```python
from build123d import *
from build123d.topology import SkipClean

# Parameters (mm, degrees)
SKETCH1_R           = 100
SKETCH1_R_2         = 50
BOSS_EXTRUDE3_DEPTH = 30
BOSS_EXTRUDE4_DEPTH = 10


with BuildPart() as part:
    # Sketch1 → Boss-Extrude3 (new body)
    # profile 1 of 16: a face of its own
    with SkipClean():  # the faces are left unmerged after this step: merging them gives an invalid solid
        with BuildSketch(Plane(origin=(0, 0, 0), x_dir=(1, 0, 0), z_dir=(0, 1, 0))):
            Circle(SKETCH1_R)
            with Locations(Location((0, 0, 0), (0, 0, 270))):
                Circle(SKETCH1_R_2, mode=Mode.SUBTRACT)
        # profile 2 of 16: a face of its own
        with BuildSketch(Plane(origin=(0, 0, 0), x_dir=(1, 0, 0), z_dir=(0, 1, 0))):
            with BuildLine():
                ThreePointArc((-15, 52.915026221), (0, 55), (15, 52.915026221))
                Line((15, 52.915026221), (15, 98.868599666))
                ThreePointArc((15, 98.868599666), (0, 100), (-15, 98.868599666))
                Line((-15, 98.868599666), (-15, 52.915026221))
            make_face()
        # profile 3 of 16: a face of its own
        with BuildSketch(Plane(origin=(0, 0, 0), x_dir=(1, 0, 0), z_dir=(0, 1, 0))):
            with BuildLine():
                ThreePointArc((-15, 47.696960071), (-7.587884964, 49.420886291), (0, 50))
                ThreePointArc((0, 50), (7.587884964, 49.420886291), (15, 47.696960071))
                Line((15, 47.696960071), (15, 52.915026221))
                ThreePointArc((15, 52.915026221), (0, 55), (-15, 52.915026221))
                Line((-15, 52.915026221), (-15, 47.696960071))
            make_face()
        # profile 4 of 16: a face of its own
        with BuildSketch(Plane(origin=(0, 0, 0), x_dir=(1, 0, 0), z_dir=(0, 1, 0))):
            with BuildLine():
                ThreePointArc((-15, 98.868599666), (0, 100), (15, 98.868599666))
                Line((15, 98.868599666), (15, 115))
                ThreePointArc((15, 115), (13.535533906, 118.535533906), (10, 120))
                Line((10, 120), (-10, 120))
                ThreePointArc((-10, 120), (-13.535533906, 118.535533906), (-15, 115))
                Line((-15, 115), (-15, 98.868599666))
            make_face()
        # profile 5 of 16: a face of its own
        with BuildSketch(Plane(origin=(0, 0, 0), x_dir=(1, 0, 0), z_dir=(0, 1, 0))):
            with BuildLine():
                ThreePointArc((-98.868599666, -15), (-100, 0), (-98.868599666, 15))
                Line((-98.868599666, 15), (-115, 15))
                ThreePointArc((-115, 15), (-118.535533906, 13.535533906), (-120, 10))
                Line((-120, 10), (-120, -10))
                ThreePointArc((-120, -10), (-118.535533906, -13.535533906), (-115, -15))
                Line((-115, -15), (-98.868599666, -15))
            make_face()
        # profile 6 of 16: a face of its own
        with BuildSketch(Plane(origin=(0, 0, 0), x_dir=(1, 0, 0), z_dir=(0, 1, 0))):
            with BuildLine():
                ThreePointArc((-52.915026221, -15), (-55, 0), (-52.915026221, 15))
                Line((-52.915026221, 15), (-98.868599666, 15))
                ThreePointArc((-98.868599666, 15), (-100, 0), (-98.868599666, -15))
                Line((-98.868599666, -15), (-52.915026221, -15))
            make_face()
        # profile 7 of 16: a face of its own
        with BuildSketch(Plane(origin=(0, 0, 0), x_dir=(1, 0, 0), z_dir=(0, 1, 0))):
            with BuildLine():
                ThreePointArc((-47.696960071, 15), (-35.355339059, 35.355339059), (-15, 47.696960071))
                Line((-15, 47.696960071), (-15, 52.915026221))
                Line((-15, 52.915026221), (-15, 98.868599666))
                ThreePointArc((-15, 98.868599666), (-70.710678119, 70.710678119), (-98.868599666, 15))
                Line((-98.868599666, 15), (-52.915026221, 15))
                Line((-52.915026221, 15), (-47.696960071, 15))
            make_face()
        # profile 8 of 16: a face of its own
        with BuildSketch(Plane(origin=(0, 0, 0), x_dir=(1, 0, 0), z_dir=(0, 1, 0))):
            with BuildLine():
                Line((-15, -52.915026221), (-15, -47.696960071))
                ThreePointArc((-15, -47.696960071), (-35.355339059, -35.355339059), (-47.696960071, -15))
                Line((-47.696960071, -15), (-52.915026221, -15))
                Line((-52.915026221, -15), (-98.868599666, -15))
                ThreePointArc((-98.868599666, -15), (-70.710678119, -70.710678119), (-15, -98.868599666))
                Line((-15, -98.868599666), (-15, -52.915026221))
            make_face()
        # profile 9 of 16: a face of its own
        with BuildSketch(Plane(origin=(0, 0, 0), x_dir=(1, 0, 0), z_dir=(0, 1, 0))):
            with BuildLine():
                ThreePointArc((15, -52.915026221), (0, -55), (-15, -52.915026221))
                Line((-15, -52.915026221), (-15, -98.868599666))
                ThreePointArc((-15, -98.868599666), (0, -100), (15, -98.868599666))
                Line((15, -98.868599666), (15, -52.915026221))
            make_face()
        # profile 10 of 16: a face of its own
        with BuildSketch(Plane(origin=(0, 0, 0), x_dir=(1, 0, 0), z_dir=(0, 1, 0))):
            with BuildLine():
                ThreePointArc((15, -98.868599666), (0, -100), (-15, -98.868599666))
                Line((-15, -98.868599666), (-15, -115))
                ThreePointArc((-15, -115), (-13.535533906, -118.535533906), (-10, -120))
                Line((-10, -120), (10, -120))
                ThreePointArc((10, -120), (13.535533906, -118.535533906), (15, -115))
                Line((15, -115), (15, -98.868599666))
            make_face()
        # profile 11 of 16: a face of its own
        with BuildSketch(Plane(origin=(0, 0, 0), x_dir=(1, 0, 0), z_dir=(0, 1, 0))):
            with BuildLine():
                ThreePointArc((47.696960071, -15), (35.355339059, -35.355339059), (15, -47.696960071))
                Line((15, -47.696960071), (15, -52.915026221))
                Line((15, -52.915026221), (15, -98.868599666))
                ThreePointArc((15, -98.868599666), (70.710678119, -70.710678119), (98.868599666, -15))
                Line((98.868599666, -15), (52.915026221, -15))
                Line((52.915026221, -15), (47.696960071, -15))
            make_face()
        # profile 12 of 16: a face of its own
        with BuildSketch(Plane(origin=(0, 0, 0), x_dir=(1, 0, 0), z_dir=(0, 1, 0))):
            with BuildLine():
                Line((98.868599666, 15), (52.915026221, 15))
                ThreePointArc((52.915026221, 15), (55, 0), (52.915026221, -15))
                Line((52.915026221, -15), (98.868599666, -15))
                ThreePointArc((98.868599666, -15), (99.71674876, -7.521304187), (100, 0))
                ThreePointArc((100, 0), (99.71674876, 7.521304187), (98.868599666, 15))
            make_face()
        # profile 13 of 16: a face of its own
        with BuildSketch(Plane(origin=(0, 0, 0), x_dir=(1, 0, 0), z_dir=(0, 1, 0))):
            with BuildLine():
                Line((115, 15), (98.868599666, 15))
                ThreePointArc((98.868599666, 15), (99.71674876, 7.521304187), (100, 0))
                ThreePointArc((100, 0), (99.71674876, -7.521304187), (98.868599666, -15))
                Line((98.868599666, -15), (115, -15))
                ThreePointArc((115, -15), (118.535533906, -13.535533906), (120, -10))
                Line((120, -10), (120, 10))
                ThreePointArc((120, 10), (118.535533906, 13.535533906), (115, 15))
            make_face()
        # profile 14 of 16: a face of its own
        with BuildSketch(Plane(origin=(0, 0, 0), x_dir=(1, 0, 0), z_dir=(0, 1, 0))):
            with BuildLine():
                Line((15, 52.915026221), (15, 47.696960071))
                ThreePointArc((15, 47.696960071), (35.355339059, 35.355339059), (47.696960071, 15))
                Line((47.696960071, 15), (52.915026221, 15))
                Line((52.915026221, 15), (98.868599666, 15))
                ThreePointArc((98.868599666, 15), (70.710678119, 70.710678119), (15, 98.868599666))
                Line((15, 98.868599666), (15, 52.915026221))
            make_face()
        # profile 15 of 16: a face of its own
        with BuildSketch(Plane(origin=(0, 0, 0), x_dir=(1, 0, 0), z_dir=(0, 1, 0))):
            with BuildLine():
                ThreePointArc((15, -47.696960071), (7.587884964, -49.420886291), (0, -50))
                ThreePointArc((0, -50), (-7.587884964, -49.420886291), (-15, -47.696960071))
                Line((-15, -47.696960071), (-15, -52.915026221))
                ThreePointArc((-15, -52.915026221), (0, -55), (15, -52.915026221))
                Line((15, -52.915026221), (15, -47.696960071))
            make_face()
        # profile 16 of 16: a face of its own
        with BuildSketch(Plane(origin=(0, 0, 0), x_dir=(1, 0, 0), z_dir=(0, 1, 0))):
            with BuildLine():
                Line((52.915026221, 15), (47.696960071, 15))
                ThreePointArc((47.696960071, 15), (49.420886291, 7.587884964), (50, 0))
                ThreePointArc((50, 0), (49.420886291, -7.587884964), (47.696960071, -15))
                Line((47.696960071, -15), (52.915026221, -15))
                ThreePointArc((52.915026221, -15), (55, 0), (52.915026221, 15))
            make_face()
        extrude(amount=BOSS_EXTRUDE3_DEPTH)

    # Sketch1<7> → Boss-Extrude4 (add)
    with SkipClean():  # the faces are left unmerged after this step: merging them gives an invalid solid
        with BuildSketch(Plane(origin=(0, 0, 0), x_dir=(1, 0, 0), z_dir=(0, 1, 0))):
            with BuildLine():
                ThreePointArc((15, 47.696960071), (7.587884964, 49.420886291), (0, 50))
                Line((0, 50), (0, -50))
                ThreePointArc((0, -50), (7.587884964, -49.420886291), (15, -47.696960071))
                ThreePointArc((15, -47.696960071), (35.355339059, -35.355339059), (47.696960071, -15))
                ThreePointArc((47.696960071, -15), (49.420886291, -7.587884964), (50, 0))
                ThreePointArc((50, 0), (49.420886291, 7.587884964), (47.696960071, 15))
                ThreePointArc((47.696960071, 15), (35.355339059, 35.355339059), (15, 47.696960071))
            make_face()
            with BuildLine():
                Line((0, -50), (0, 50))
                ThreePointArc((0, 50), (-7.587884964, 49.420886291), (-15, 47.696960071))
                ThreePointArc((-15, 47.696960071), (-35.355339059, 35.355339059), (-47.696960071, 15))
                ThreePointArc((-47.696960071, 15), (-50, 0), (-47.696960071, -15))
                ThreePointArc((-47.696960071, -15), (-35.355339059, -35.355339059), (-15, -47.696960071))
                ThreePointArc((-15, -47.696960071), (-7.587884964, -49.420886291), (0, -50))
            make_face()
        extrude(amount=BOSS_EXTRUDE4_DEPTH)


solid = part.part
```
Read the model definition and answer for the solid it produces. Units are mm, in the model's axes. A direction names the side the tool comes from. Coordinates: 2 decimals unless noted, no trailing zeros. Write each loop counter-clockwise with the first axis right and the second up, starting at its lowest first coordinate (ties: lowest second). Pieces come first, ordered by that corner, then holes. Notation, with made-up numbers: (-14.5, 46) -> (10.5, 46) arc R30 ccw to (10.5, 75) -> close; hole circle Ø5 at (81.25, -19.5). An arc over 180 degrees is marked (long way). Return JSON: item names as keys, results as strings.
1. A cutting plane is placed at C-C (x = 0). Determine the outline of the cut face in (y, z).
Found:
{"outline": "(0, -120) -> (30, -120) -> (30, -50) -> (10, -50) -> (10, 50) -> (30, 50) -> (30, 120) -> (0, 120) -> close"}
2. Find the intervals of material crossed by line 1 along Z through (x, y) = (0, 19.75); line 2 along Y through (x, z) = (25.5, -9), in increasing order. Write a range as from..to.
Found:
{"line 1": "-120..-50, 50..120", "line 2": "0..10"}
3. A cutting plane is placed at A-A (y = 13.75). Determine the outline of the cut face in (x, z).
Found:
{"outline": "(-120, -10) arc R5 ccw to (-115, -15) -> (-98.87, -15) arc R100 ccw to (-15, -98.87) -> (-15, -115) arc R5 ccw to (-10, -120) -> (10, -120) arc R5 ccw to (15, -115) -> (15, -98.87) arc R100 ccw to (98.87, -15) -> (115, -15) arc R5 ccw to (120, -10) -> (120, 10) arc R5 ccw to (115, 15) -> (98.87, 15) arc R100 ccw to (15, 98.87) -> (15, 115) arc R5 ccw to (10, 120) -> (-10, 120) arc R5 ccw to (-15, 115) -> (-15, 98.87) arc R100 ccw to (-98.87, 15) -> (-115, 15) arc R5 ccw to (-120, 10) -> close; hole circle Ø100 at (0, 0)"}
4. A cutting plane is placed at B-B (z = 7). Determine the outline of the cut face in (x, y).
Found:
{"outline": "(-120, 0) -> (120, 0) -> (120, 30) -> (49.51, 30) -> (49.51, 10) -> (-49.51, 10) -> (-49.51, 30) -> (-120, 30) -> close"}
5. A cutting plane is placed at D-D (z = 81). Determine the outline of the cut face in (x, y).
Found:
{"outline": "(-58.64, 0) -> (58.64, 0) -> (58.64, 30) -> (-58.64, 30) -> close"}
6. A tool of negligible diameter and unlimited length cuts with its end or side. For faces 1 (the face through (107, 15, 15)), 2 (the face through (15, 15, -107)), 3 (the face through (-107, 15, -15)), 4 (the face through (-107, 15, 15)), from which of +Z, -Z, +X, -X, +Y, -Y can it reach the whole face along a straight path? Write none if from no direction.
Found:
{"face 1": "+Z, +X, +Y, -Y", "face 2": "-Z, +X, +Y, -Y", "face 3": "-Z, -X, +Y, -Y", "face 4": "+Z, -X, +Y, -Y"}
7. Each of these flat-tipped pins is pushed along its axis until it touches: P1, Ø3, axis at x = -18.5, z = 3, coming from the +Y side; P2, Ø17.5, axis at y = 12, z = 108, coming from the -X side; P3, Ø1, axis at x = 90, y = 21, coming from the +Z side; P4, Ø10, axis at x = -33, z = -26.5, coming from the -Y side. Where does it stop, or does it pass through?
Found:
{"P1": "y = 10", "P2": "x = -15", "P3": "z = 44.61", "P4": "y = 0"}
8. Determine the mould class of faces 5 (the face through (0, 15, -120)), 6 (the face through (-1, 10, -1)), 7 (the face through (-15, 15, -107)), 8 (the face through (15, 15, 107)) for opening direction X: pulls with the +X half, pulls with the -X half, needs draft (parallel to the pull), parting line crosses it, or undercut.
Found:
{"face 5": "needs draft", "face 6": "undercut", "face 7": "pulls with the -X half", "face 8": "pulls with the +X half"}
